Source: CAD feature listing. Evaluate the final solid. Frame: model axes, mm. A direction names the side the tool comes from. Give positions to 0.01 mm unless a question says otherwise; leave off trailing zeros. Loops run counter-clockwise (first coordinate to the right, second up) from the corner with the lowest first, then second, coordinate; pieces in that order, holes last.
from build123d import *

# Parameters (mm, degrees)
BOSS_EXTRUDE1_DEPTH        = 25.4
SKETCH2_R                  = 4.1671875
CUT_EXTRUDE1_DEPTH         = 43.715256349
F_8_0_199_DIAMETER_HOLE1_D = 5.0546


with BuildPart() as part:
    # Sketch1 → Boss-Extrude1 (new body)
    with BuildSketch(Plane.XY):
        Polygon((-14.2875, 9.525), (-14.2875, -9.525), (-11.1125, -9.525), (-11.1125, 9.525), (11.1125, 9.525), (11.1125, -9.525), (14.2875, -9.525), (14.2875, 19.05), (-39.6875, 19.05), (-39.6875, 9.525), align=None)
    extrude(amount=BOSS_EXTRUDE1_DEPTH)

    # Sketch2 → Cut-Extrude1 (cut, through all)
    with BuildSketch(Plane.ZY.offset(14.2875)):
        with Locations((12.7, -3.96875)):
            Circle(SKETCH2_R)
    extrude(amount=-CUT_EXTRUDE1_DEPTH, mode=Mode.SUBTRACT)

    # #8 (0.199) Diameter Hole1 (through all)
    with Locations(Plane(origin=(0, 19.05, 0), x_dir=(1, 0, 0), z_dir=(0, 1, 0))):
        with Locations((-34.3296875, -12.7), (5.7546875, -12.7)):
            Hole(F_8_0_199_DIAMETER_HOLE1_D / 2)


solid = part.part
1) Ray query, probe 1 along X at (y, z) = (11.5, 12.7); probe 2 along Y at (x, z) = (-13.4, 12.7) (3 decimals); probe 3 along X at (y, z) = (8.75, 23.5). Return the intervals inside material, ascending.
Checks:
probe 1: x = -39.69 to -36.86, -31.8 to 3.23, 8.28 to 14.29
probe 2: y = -9.525 to -8.136, 0.198 to 19.05
probe 3: x = -14.29 to -11.11, 11.11 to 14.29
2) Contact query for flat-ended pins moving along their axis: P1, Ø12.5, axis at x = -30.5, z = 7.5, coming from the -Y side (3 decimals); P2, Ø15, axis at y = -1, z = 9, coming from the -X side; P3, Ø6.5, axis at y = -3.97, z = 12.7, coming from the -X side. Output: stop coordinate, or through.
Checks:
P1: stops at y = 9.525
P2: stops at x = -14.29
P3: passes through
3) Pull-direction query (Z, two-part tool) for faces 1 (the cylindrical face through (4.588, 14.221, 14.942)), 2 (the flat face through (-13, 11, 0)), 3 (the flat face through (-27, 9.525, 13)), 4 (the flat face through (-13, 11, 25.4)); classes: released by +Z, released by -Z, zero draft, split by the parting line, or undercut.
Checks:
face 1: undercut
face 2: released by -Z
face 3: zero draft
face 4: released by +Z
4) Reachability of faces 5 (the flat face through (-11.112, 2, 13)), 6 (the flat face through (14.288, 5, 13)), 7 (the flat face through (-14.288, 2, 13)) from +Z, -Z, +X, -X, +Y, -Y: full face, straight path, thin tool, end or side. Return the list, or none.
Checks:
face 5: +Z, -Z, -Y
face 6: +Z, -Z, +X, +Y, -Y
face 7: +Z, -Z, -X, -Y
5) Cut plane C-C (x = -35). Return loops of the section in (y, z) (3 decimals).
Checks:
outline: (9.525, 0) - (19.05, 0) - (19.05, 10.263) - (9.525, 10.263) - close; (9.525, 15.137) - (19.05, 15.137) - (19.05, 25.4) - (9.525, 25.4) - close
6) Cut plane A-A (z = 12.7). State how many separate pieces and enclosed holes the cut face has, and give its area (3 significant figures).
Checks:
separate pieces: 5
enclosed holes: 0
area: 486 mm2
7) Cut plane D-D (y = -1.5). Return loops of the section in (x, z), and give its area (3 significant figures).
Checks:
outline: (-14.29, 0) - (-11.11, 0) - (-11.11, 9.34) - (-14.29, 9.34) - close; (-14.29, 16.06) - (-11.11, 16.06) - (-11.11, 25.4) - (-14.29, 25.4) - close; (11.11, 0) - (14.29, 0) - (14.29, 9.34) - (11.11, 9.34) - close; (11.11, 16.06) - (14.29, 16.06) - (14.29, 25.4) - (11.11, 25.4) - close
area: 119 mm2
8) Cut plane B-B (y = 7). Return loops of the section in (x, z), and give its area (3 significant figures).
Checks:
outline: (-14.29, 0) - (-11.11, 0) - (-11.11, 25.4) - (-14.29, 25.4) - close; (11.11, 0) - (14.29, 0) - (14.29, 25.4) - (11.11, 25.4) - close
area: 161 mm2
